The listing builds one solid part. Answer for the finished solid, in the listing's coordinates (mm). A direction names the side the tool comes from. Round coordinates to 2 decimals unless told otherwise and drop trailing zeros. Loops run counter-clockwise (first coordinate to the right, second up) from the corner with the lowest first, then second, coordinate; pieces in that order, holes last. Notation, with made-up numbers: (-1.5, 10) - (56.5, 10) arc R18 ccw to (56.5, 24) - close; hole circle Ø8 at (32, 43.25). An arc over 180 degrees is marked (long way). One line per item, written item: value.
```python
from build123d import *

# Parameters (mm, degrees)
SKETCH1_R           = 1.5
BOSS_EXTRUDE1_DEPTH = 5
SKETCH2_R           = 7
BOSS_EXTRUDE2_DEPTH = 5
FILLET1_R           = 10
FILLET2_R           = 3


with BuildPart() as part:
    # Sketch1 → Boss-Extrude1 (new body)
    with BuildSketch(Plane(origin=(0, 0, 0), x_dir=(1, 0, 0), z_dir=(0, 1, 0))):
        Polygon((-20, 20), (-20, -20), (20, -20), (20, 20), (20, 30), (-20, 30), align=None)
        with Locations(Location((14, 0, 0), (0, 0, 270))):
            Circle(SKETCH1_R, mode=Mode.SUBTRACT)
        with Locations(Location((-14, 0, 0), (0, 0, 270))):
            Circle(SKETCH1_R, mode=Mode.SUBTRACT)
        with BuildLine():
            Line((-2.645751311, -3), (2.645751311, -3))
            ThreePointArc((2.645751311, -3), (0, 4), (-2.645751311, -3))
        make_face(mode=Mode.SUBTRACT)
    extrude(amount=BOSS_EXTRUDE1_DEPTH)

    # Sketch2 → Boss-Extrude2 (add)
    with BuildSketch(Plane(origin=(0, 5, 0), x_dir=(1, 0, 0), z_dir=(0, 1, 0))):
        with Locations(Location((0, 0, 0), (0, 0, 270))):
            Circle(SKETCH2_R)
        with BuildLine():
            ThreePointArc((-2.645751311, -3), (0, 4), (2.645751311, -3))
            Line((2.645751311, -3), (-2.645751311, -3))
        make_face(mode=Mode.SUBTRACT)
    extrude(amount=BOSS_EXTRUDE2_DEPTH)

    # Fillet1
    fillet1_edges = [part.edges().sort_by_distance(p)[0] for p in [
        (20, 2.5, 20),
        (-20, 2.5, 20),
    ]]
    fillet(fillet1_edges, radius=FILLET1_R)

    # Fillet2
    fillet2_edges = [part.edges().sort_by_distance(p)[0] for p in [
        (0, 5, -7),
    ]]
    fillet(fillet2_edges, radius=FILLET2_R)


solid = part.part
```
1) For faces 1 (the flat face through (0, 2, -30)), 2 (the cylindrical face through (-6.834, 8.986, -1.517)), 3 (the flat face through (0, 5, 3)), determine the directions among +Z, -Z, +X, -X, +Y, -Y from which every point of the face is accessible in a straight line to the end or side of a thin tool.
Final values:
face 1: -Z, +X, -X, +Y, -Y
face 2: +Y
face 3: +Y, -Y
2) A cutting plane is placed at B-B on y = 4.25. Give the vertices of the cut face in (x, z).
Final values:
outline: (-20, -30) - (20, -30) - (20, 10) arc R10 ccw to (10, 20) - (-10, 20) arc R10 ccw to (-20, 10) - close; hole circle Ø3 at (-14, 0); hole (-2.65, 3) arc R4 ccw (long way) to (2.65, 3) - close; hole circle Ø3 at (14, 0)
3) Consider L1, parallel to X at y = 3.55, z = 0; L2, parallel to Y at x = 5, z = 11; L3, parallel to X at y = 7.9, z = 0. Determine where each line is inside the solid, lowest interval first.
Final values:
L1: -20 to -15.5, -12.5 to -4, 4 to 12.5, 15.5 to 20
L2: 0 to 5
L3: -7 to -4, 4 to 7
4) A cutting plane is placed at C-C on z = -22.5. Give the vertices of the cut face in (x, y).
Final values:
outline: (-20, 0) - (20, 0) - (20, 5) - (-20, 5) - close
5) For a pull along X with two mould halves and no side action, classify faces 4 (the flat face through (-3, 10, 3)), 5 (the flat face through (-20, 2, -10)), 6 (the cylindrical face through (14.45, 2.46, 1.43)) as released by +X, released by -X, zero draft, split by the parting line, or undercut.
Final values:
face 4: zero draft
face 5: released by -X
face 6: undercut
6) A cutting plane is placed at D-D on y = 7.25. Give the vertices of the cut face in (x, z), and give its area (3 significant figures).
Final values:
outline: circle Ø14.19 at (0, 0); hole (-2.65, 3) arc R4 ccw (long way) to (2.65, 3) - close
area: 112 mm2
7) Each of these flat-tipped pins is pushed along its axis until it touches: pin 1 Ø2.5 at (x, z) = (-14, 0) entering from -Y; pin 2 Ø3 at (x, y) = (0.5, 8.5) entering from -Z. Where does it stop, or does it pass through?
Final values:
pin 1: through
pin 2: z = -7.16
8) A cutting plane is placed at A-A on x = 0. Give the vertices of the cut face in (y, z).
Final values:
outline: (0, -30) - (5, -30) - (5, -10) arc R3 cw to (8, -7) - (10, -7) - (10, -4) - (0, -4) - close; (0, 3) - (10, 3) - (10, 7) - (8, 7) arc R3 cw to (5, 10) - (5, 20) - (0, 20) - close
